Geometry check sheet. Reference: the model listing, model coordinates, mm. Give positions to 0.01 mm unless a question says otherwise; leave off trailing zeros. Write each loop counter-clockwise with the first axis right and the second up, starting at its lowest first coordinate (ties: lowest second). Pieces come first, ordered by that corner, then holes. Notation, with made-up numbers: M 79,-27 L 88,-27 A13 ccw 88,-5 Z; hole C 89,34.25 d7. An arc over 180 degrees is marked long. One line per item, written item: value. Start each with the question number.
1. Gauge pin test, flat ends, axial feed: pin 1 (4 mm diameter, centred on y = 2, z = 58.5, fed in from +X); pin 2 (4 mm diameter, centred on x = 180.5, y = 4, fed in from -Z); pin 3 (3 mm diameter, centred on x = 18.5, y = 2, fed in from -Z). Record the tip position at first contact, or that the pin passes through.
2. Cross-section at B-B on x = -12.5. Record the cut outline in (y, z), then the cut area to 3 significant figures.
3. Cross-section at D-D on z = 61. Record the cut outline in (x, y).
4. Scan lines: line 1 (Z direction, x = 228.6, y = 4.5); line 2 (Z direction, x = 177.8, y = 3.75); line 3 (Z direction, x = 75, y = 4.75). Record each from-to range of solid material in increasing order.
5. Cross-section at A-A on y = 1.25. Count the separate pieces of the cut face and the enclosed holes in it, then the cut area to 3 significant figures.
6. Cross-section at C-C on z = -25.4. Record the cut outline in (x, y), then the cut area to 3 significant figures.
from build123d import *

# Parameters (mm, degrees)
BOSS_EXTRUDE1_DEPTH     = 7.9375
SKETCH21_R              = 22.1615
SKETCH21_R_2            = 2.0193
CUT_EXTRUDE2_DEPTH      = 253.811910138
FILLET1_R               = 7.62
L_0_29_DIAMETER_HOLE1_D = 7.366


with BuildPart() as part:
    # Sketch1 → Boss-Extrude1 (new body)
    with BuildSketch(Plane(origin=(0, 0, 0), x_dir=(1, 0, 0), z_dir=(0, 1, 0))):
        with BuildLine():
            Line((241.3, -44.45), (60.409978491, -44.45))
            ThreePointArc((60.409978491, -44.45), (-75.00112, 0), (60.409978491, 44.45))
            Line((60.409978491, 44.45), (241.3, 44.45))
            Line((241.3, 44.45), (241.3, -44.45))
        make_face()
    extrude(amount=BOSS_EXTRUDE1_DEPTH)

    # Sketch21 → Cut-Extrude2 (cut, through all)
    with BuildSketch(Plane(origin=(0, 7.9375, 0), x_dir=(1, 0, 0), z_dir=(0, 1, 0))):
        with Locations(Location((0, 0, 0), (0, 0, 270))):
            Circle(SKETCH21_R)
        with Locations(Location((0, 33.02, 0), (0, 0, 270))):
            Circle(SKETCH21_R_2)
        with Locations(Location((-33.02, 0, 0), (0, 0, 270))):
            Circle(SKETCH21_R_2)
        with Locations(Location((0, -33.02, 0), (0, 0, 270))):
            Circle(SKETCH21_R_2)
        with Locations(Location((33.02, 0, 0), (0, 0, 270))):
            Circle(SKETCH21_R_2)
        with Locations(Location((25.4, -25.4, 0), (0, 0, 270))):
            Circle(SKETCH21_R_2)
    extrude(amount=-CUT_EXTRUDE2_DEPTH, mode=Mode.SUBTRACT)

    # Fillet1
    fillet1_edges = [part.edges().sort_by_distance(p)[0] for p in [
        (60.409978491, 3.96875, -44.45),
        (241.3, 3.96875, -44.45),
        (241.3, 3.96875, 44.45),
        (60.409978491, 3.96875, 44.45),
    ]]
    fillet(fillet1_edges, radius=FILLET1_R)

    # L (0.29) Diameter Hole1 (through all)
    with Locations(Plane(origin=(0, 7.9375, 0), x_dir=(1, 0, 0), z_dir=(0, 1, 0))):
        with Locations((228.6, 25.4), (228.6, -25.4), (203.2, 0), (177.8, 0)):
            Hole(L_0_29_DIAMETER_HOLE1_D / 2)


solid = part.part
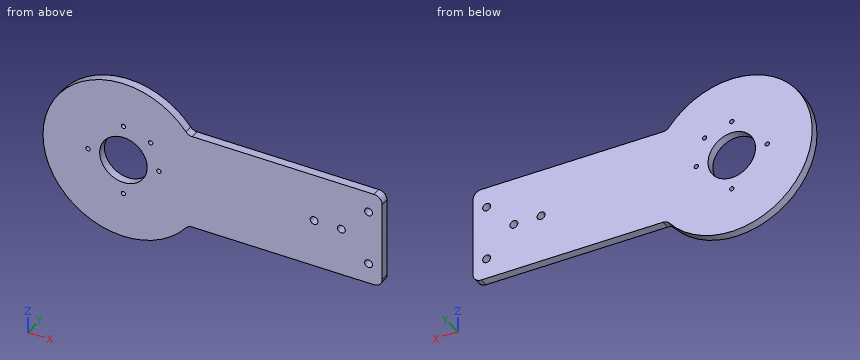
Report:
1. pin 1: stops at x = 49.32
1. pin 2: stops at z = -44.45
1. pin 3: stops at z = -73.05
2. outline: M 0,-73.95 L 7.94,-73.95 L 7.94,-18.3 L 0,-18.3 Z; M 0,18.3 L 7.94,18.3 L 7.94,73.95 L 0,73.95 Z
2. area: 883 mm^2
3. outline: M -43.64,0 L 43.64,0 L 43.64,7.94 L -43.64,7.94 Z
4. line 1: z = -44.45 to -29.08, -21.72 to 21.72, 29.08 to 44.45
4. line 2: z = -44.45 to -3.68, 3.68 to 44.45
4. line 3: z = -44.45 to 44.45
5. separate pieces: 1
5. enclosed holes: 10
5. area: 31,100 mm^2
6. outline: M -70.57,0 L 224.92,0 L 224.92,7.94 L -70.57,7.94 Z; M 232.28,0 L 241.3,0 L 241.3,7.94 L 232.28,7.94 Z
6. area: 2,420 mm^2
